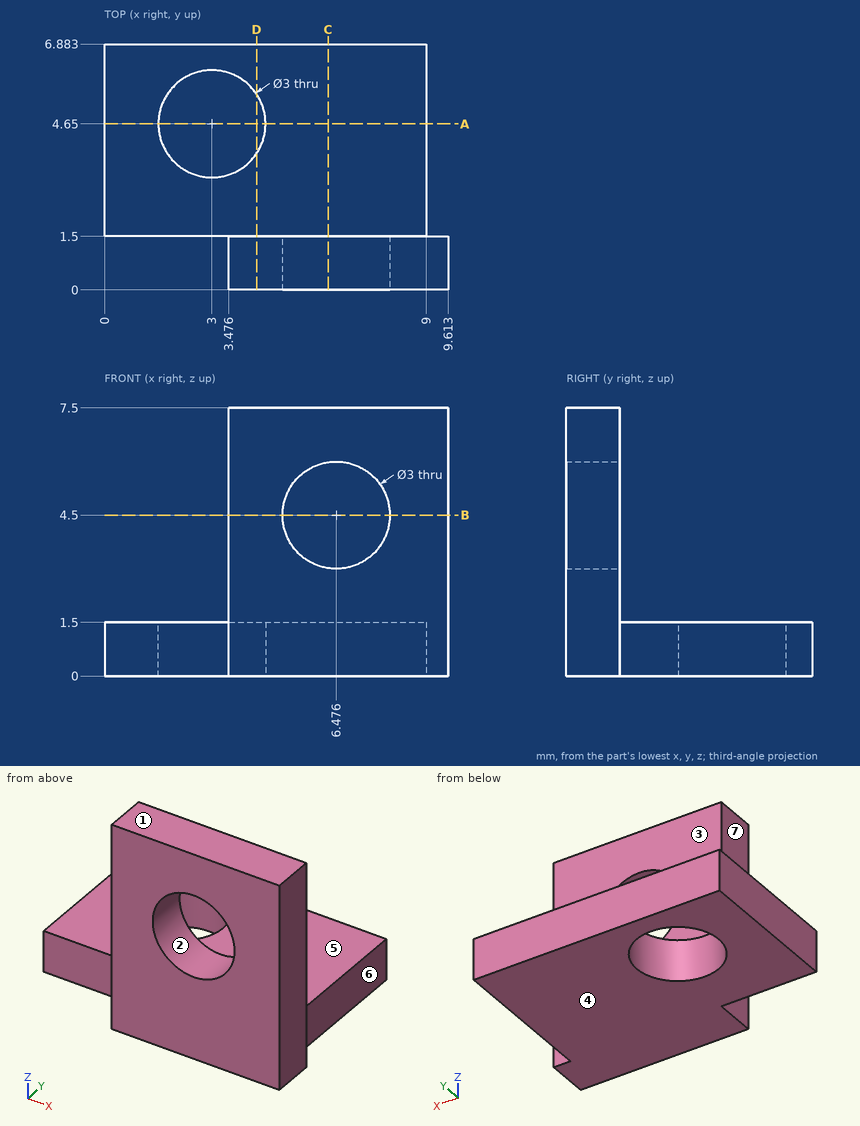
Print and shaded views of the part. All mm, measured from the part's lowest x, y and z. A direction names the side the tool comes from. Coordinates: 2 decimals unless noted, no trailing zeros. Order: outer loops, then holes, each group sorted by start corner. A loop starts at its lowest first (then second) coordinate and runs counter-clockwise, first axis right, second up. Notation, with made-up numbers: M 85.25,-23 L 124.25,-23 A34 ccw 124.25,12 Z; hole C -35,12 d11. An arc over 180 degrees is marked long. One line per question, with ' | ' between items. Start each with the question number.
Q1. Saw through at C-C (x = 6.25). List the corners of the cut face in (y, z), then the cut area to 3 significant figures.
Q2. Saw through at A-A (y = 4.65). List the corners of the cut face in (x, z).
Q3. Saw through at B-B (z = 4.5). List the corners of the cut face in (x, y) (1 decimal).
Q4. Two-plate mould, pull along Z, no slides. Class the marked faces 1, 2, 3 and 4: +Z half, -Z half, draft (parallel to the pull), parting line (faces both ways), or undercut.
Q5. Saw through at D-D (x = 4.25). List the corners of the cut face in (y, z).
Q6. Flat gauge pins, fed straight in: pin 1 Ø1.6 at (x, z) = (1, 0.5) entering from -Y; pin 2 Ø3 at (x, z) = (3.5, 5.5) entering from +Y; pin 3 Ø1.2 at (y, z) = (3.5, 0.5) entering from +X. Where does each tip first touch, or does it go through?
Q7. Probe L1, parallel to X at y = 1.1, z = 4.5 (1 decimal); L2, parallel to Y at x = 3, z = 0.75; L3, parallel to Z at x = 1, y = 4.5. List the from-to ranges inside material, lowest first. Write a range as from..to.
Q8. 3-axis set-ups, long thin cutter, end or side, ignore diameter. For the marked faces 5, 6 and 7: which of +Z, -Z, +X, -X, +Y, -Y reach the whole face in a straight line?
Check values:
1) outline: M 0,0 L 6.88,0 L 6.88,1.5 L 1.5,1.5 L 1.5,3.02 L 0,3.02 Z; M 0,5.98 L 1.5,5.98 L 1.5,7.5 L 0,7.5 Z | area: 14.9 mm2
2) outline: M 0,0 L 1.5,0 L 1.5,1.5 L 0,1.5 Z; M 4.5,0 L 9,0 L 9,1.5 L 4.5,1.5 Z
3) outline: M 3.5,0 L 5,0 L 5,1.5 L 3.5,1.5 Z; M 8,0 L 9.6,0 L 9.6,1.5 L 8,1.5 Z
4) face 1: +Z half | face 2: undercut | face 3: draft | face 4: -Z half
5) outline: M 0,0 L 3.82,0 L 3.82,1.5 L 1.5,1.5 L 1.5,7.5 L 0,7.5 Z; M 5.48,0 L 6.88,0 L 6.88,1.5 L 5.48,1.5 Z
6) pin 1: stops at y = 1.5 | pin 2: stops at y = 1.5 | pin 3: stops at x = 9
7) L1: x = 3.5..5, 8..9.6 | L2: y = 1.5..3.15, 6.15..6.88 | L3: z = 0..1.5
8) face 5: +Z, +X, -X, +Y | face 6: +Z, -Z, +X, +Y | face 7: +Z, -Z, -X, -Y
